Can you work these out from the drawing? Everything is in mm from the part's minimum corner. A direction names the side the tool comes from. Give positions to 0.01 mm unless a question says otherwise; leave off trailing zeros. Write each loop counter-clockwise with the first axis right and the second up, starting at its lowest first coordinate (ties: lowest second). Pieces come first, ordered by that corner, then holes. Notation, with made-up numbers: (0.5, 47) - (50.5, 47) arc R18 cw to (50.5, 71) - close; hole circle Ø7 at (83, 20.5). An arc over 180 degrees is marked (long way). Use a Markdown table: item, result.
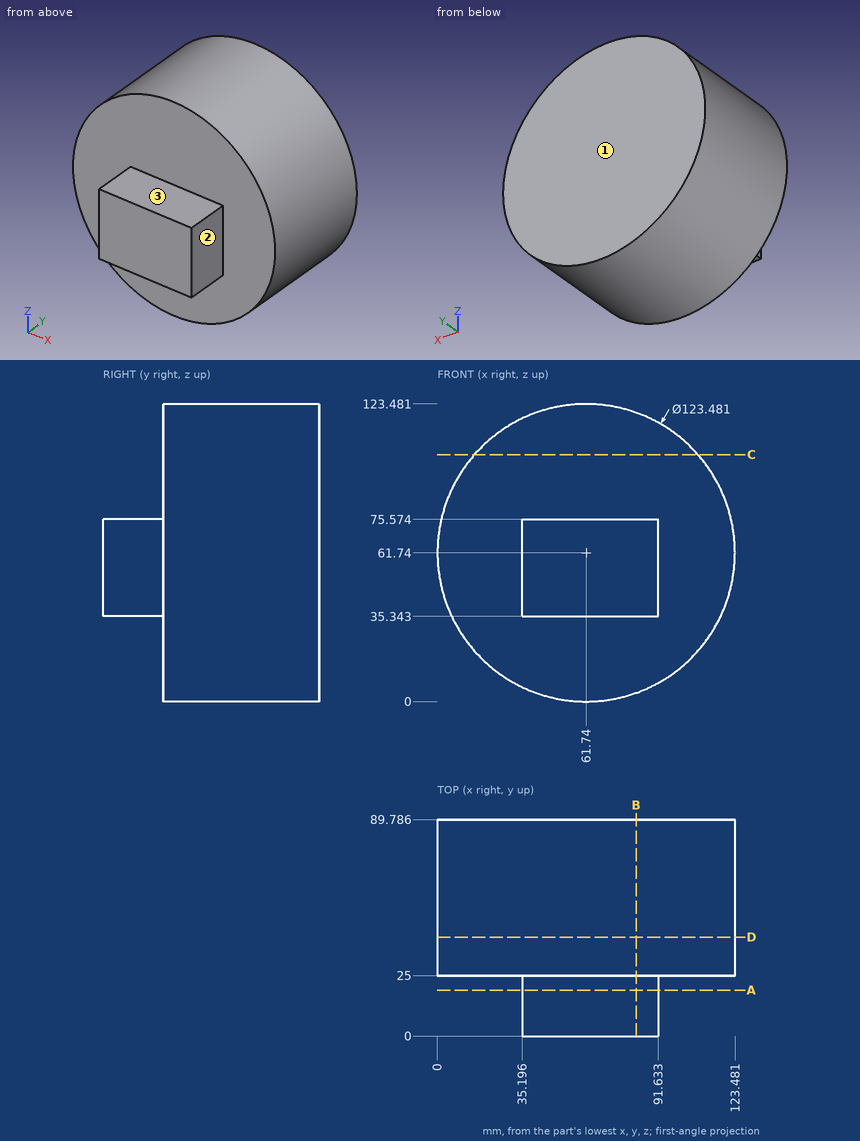
Item 1: If we section it at B-B, the plane x = 82.5: Write out the boundary of the cut face in (y, z) (1 decimal), plus the area to 3 significant figures.
Values:
| item | result |
|---|---|
| outline | (0, 35.3) - (25, 35.3) - (25, 3.6) - (89.8, 3.6) - (89.8, 119.9) - (25, 119.9) - (25, 75.6) - (0, 75.6) - close |
| area | 8,540 mm2 |
Item 2: If we section it at A-A, the plane y = 19: Write out the boundary of the cut face in (x, z) (1 decimal).
Values:
| item | result |
|---|---|
| outline | (35.2, 35.3) - (91.6, 35.3) - (91.6, 75.6) - (35.2, 75.6) - close |
Item 3: If we section it at D-D, the plane y = 41: Write out the boundary of the cut face in (x, z).
Values:
| item | result |
|---|---|
| outline | circle Ø123.48 at (61.74, 61.74) |
Item 4: For the marked faces 1, 2 and 3, which set-ups out of +Z, -Z, +X, -X, +Y, -Y let a thin tool reach every point of the face, with its end or its side?
Values:
| item | result |
|---|---|
| face 1 | +Z, -Z, +X, -X, +Y |
| face 2 | +Z, -Z, +X, -Y |
| face 3 | +Z, +X, -X, -Y |
Item 5: Will these pins go through, and if not, where does the flat tip stop? pin 1 Ø10 at (y, z) = (67, 67) entering from +X; pin 2 Ø1.5 at (x, z) = (105.5, 91) entering from -Y; pin 3 Ø1.5 at (y, z) = (38.5, 57.5) entering from +X; pin 4 Ø12 at (x, z) = (86.5, 70.5) entering from -Y.
Values:
| item | result |
|---|---|
| pin 1 | stops at x = 123.48 |
| pin 2 | stops at y = 25 |
| pin 3 | stops at x = 123.38 |
| pin 4 | stops at y = 0 |
Item 6: If we section it at C-C, the plane z = 102.5: Write out the boundary of the cut face in (x, y) (1 decimal), plus the area to 3 significant figures.
Values:
| item | result |
|---|---|
| outline | (15.4, 25) - (108.1, 25) - (108.1, 89.8) - (15.4, 89.8) - close |
| area | 6,010 mm2 |
Item 7: I need wall thicknesses on line 1 along Y through (x, z) = (107, 31.5); line 2 along Z through (x, y) = (61, 55) (1 decimal); line 3 along X through (y, z) = (66, 62). Which ranges of each line are inside material? Lowest first, please. Write a range as [from, to].
Values:
| item | result |
|---|---|
| line 1 | y = [25, 89.79] |
| line 2 | z = [0, 123.5] |
| line 3 | x = [0, 123.48] |
